Could you check a few things on this model? Use its own coordinates, in mm. Face numbers are marked on the shaded views. Round coordinates to 2 decimals unless told otherwise and drop trailing zeros. Loops run counter-clockwise (first coordinate to the right, second up) from the corner with the lowest first, then second, coordinate; pieces in that order, holes last. Notation, with made-up numbers: (84, 67.5) -> (127, 67.5) arc R28 ccw to (127, 96.5) -> close; hole circle Ø4 at (68, 55.5). An arc over 180 degrees is marked (long way). Write each question's results on one line, items separated by ' | '.
from build123d import *

# Parameters (mm, degrees)
F1_DEPTH = 5
F2_DEPTH = 7
F3_DEPTH = 1


with BuildPart() as f1:
    # F0 (on Top) → F1 (new body)
    with BuildSketch(Plane.XY):
        with BuildLine():
            Line((-12.5, -50), (0, -50))
            Line((0, -50), (0, -45))
            Line((0, -45), (-6.5, -45))
            ThreePointArc((-6.5, -45), (-8.2071067812, -45.7071067812), (-7.5, -44))
            Line((-7.5, -44), (-7.5, -35.9886))
            ThreePointArc((-7.5, -35.9886), (-8.2071067812, -34.2814932188), (-6.5, -34.9886))
            Line((-6.5, -34.9886), (0, -34.9886))
            Line((0, -34.9886), (0, -14.9886))
            Line((0, -14.9886), (-7.5, -14.9886))
            Line((-7.5, -14.9886), (-7.5, -9.9886))
            Line((-7.5, -9.9886), (0, -9.9886))
            Line((0, -9.9886), (0, 0.0114))
            Line((0, 0.0114), (-7.5, 0.0114))
            Line((-7.5, 0.0114), (-7.5, 5.0114))
            Line((-7.5, 5.0114), (0, 5.0114))
            Line((0, 5.0114), (0, 15.0114))
            Line((0, 15.0114), (-7.5, 15.0114))
            Line((-7.5, 15.0114), (-7.5, 20.0114))
            Line((-7.5, 20.0114), (0, 20.0114))
            Line((0, 20.0114), (0, 34.3023235092))
            ThreePointArc((0, 34.3023235092), (-5, 39.3023235092), (0, 44.3023235092))
            Line((0, 44.3023235092), (0, 50))
            Line((0, 50), (-12.5, 50))
            Line((-12.5, 50), (-12.5, -50))
        make_face()
        with BuildLine():
            Line((0, -50), (12.5, -50))
            Line((12.5, -50), (12.5, 50))
            Line((12.5, 50), (0, 50))
            Line((0, 50), (0, 44.3023235092))
            ThreePointArc((0, 44.3023235092), (3.5355339059, 42.8378574152), (5, 39.3023235092))
            ThreePointArc((5, 39.3023235092), (3.5355339059, 35.7667896033), (0, 34.3023235092))
            Line((0, 34.3023235092), (0, 20.0114))
            Line((0, 20.0114), (7.5, 20.0114))
            Line((7.5, 20.0114), (7.5, 15.0114))
            Line((7.5, 15.0114), (0, 15.0114))
            Line((0, 15.0114), (0, 5.0114))
            Line((0, 5.0114), (7.5, 5.0114))
            Line((7.5, 5.0114), (7.5, 0.0114))
            Line((7.5, 0.0114), (0, 0.0114))
            Line((0, 0.0114), (0, -9.9886))
            Line((0, -9.9886), (7.5, -9.9886))
            Line((7.5, -9.9886), (7.5, -14.9886))
            Line((7.5, -14.9886), (0, -14.9886))
            Line((0, -14.9886), (0, -34.9886))
            Line((0, -34.9886), (6.5, -34.9886))
            ThreePointArc((6.5, -34.9886), (7.5, -33.9886), (8.5, -34.9886))
            ThreePointArc((8.5, -34.9886), (8.2071067812, -35.6957067812), (7.5, -35.9886))
            Line((7.5, -35.9886), (7.5, -44))
            ThreePointArc((7.5, -44), (8.2071067812, -44.2928932188), (8.5, -45))
            ThreePointArc((8.5, -45), (7.5, -46), (6.5, -45))
            Line((6.5, -45), (0, -45))
            Line((0, -45), (0, -50))
        make_face()
        with BuildLine():
            Line((0, -34.9886), (0, -45))
            Line((0, -45), (6.5, -45))
            ThreePointArc((6.5, -45), (6.7928932188, -44.2928932188), (7.5, -44))
            Line((7.5, -44), (7.5, -35.9886))
            ThreePointArc((7.5, -35.9886), (6.7928932188, -35.6957067812), (6.5, -34.9886))
            Line((6.5, -34.9886), (0, -34.9886))
        make_face()
        with BuildLine():
            Line((-6.5, -45), (0, -45))
            Line((0, -45), (0, -34.9886))
            Line((0, -34.9886), (-6.5, -34.9886))
            ThreePointArc((-6.5, -34.9886), (-6.7928932188, -35.6957067812), (-7.5, -35.9886))
            Line((-7.5, -35.9886), (-7.5, -44))
            ThreePointArc((-7.5, -44), (-6.7928932188, -44.2928932188), (-6.5, -45))
        make_face()
    extrude(amount=F1_DEPTH)

    # F0 (on Top) → F2 (join)
    with BuildSketch(Plane.XY):
        with BuildLine():
            Line((0, 42.3023235092), (0, 44.3023235092))
            ThreePointArc((0, 44.3023235092), (-5, 39.3023235092), (0, 34.3023235092))
            Line((0, 34.3023235092), (0, 36.3023235092))
            ThreePointArc((0, 36.3023235092), (-3, 39.3023235092), (0, 42.3023235092))
        make_face()
        with BuildLine():
            ThreePointArc((5, 39.3023235092), (3.5355339059, 42.8378574152), (0, 44.3023235092))
            Line((0, 44.3023235092), (0, 42.3023235092))
            ThreePointArc((0, 42.3023235092), (2.1213203436, 41.4236438528), (3, 39.3023235092))
            ThreePointArc((3, 39.3023235092), (2.1213203436, 37.1810031657), (0, 36.3023235092))
            Line((0, 36.3023235092), (0, 34.3023235092))
            ThreePointArc((0, 34.3023235092), (3.5355339059, 35.7667896033), (5, 39.3023235092))
        make_face()
    extrude(amount=F2_DEPTH)

    # F0 (on Top) → F3 (join)
    with BuildSketch(Plane.XY):
        with BuildLine():
            Line((0, 41.8023235092), (0, 42.3023235092))
            ThreePointArc((0, 42.3023235092), (-3, 39.3023235092), (0, 36.3023235092))
            Line((0, 36.3023235092), (0, 36.8023235092))
            ThreePointArc((0, 36.8023235092), (-2.5, 39.3023235092), (0, 41.8023235092))
        make_face()
        with BuildLine():
            ThreePointArc((3, 39.3023235092), (2.1213203436, 41.4236438528), (0, 42.3023235092))
            Line((0, 42.3023235092), (0, 41.8023235092))
            ThreePointArc((0, 41.8023235092), (1.767766953, 41.0700904622), (2.5, 39.3023235092))
            ThreePointArc((2.5, 39.3023235092), (1.767766953, 37.5345565563), (0, 36.8023235092))
            Line((0, 36.8023235092), (0, 36.3023235092))
            ThreePointArc((0, 36.3023235092), (2.1213203436, 37.1810031657), (3, 39.3023235092))
        make_face()
    extrude(amount=F3_DEPTH)


solid = f1.part
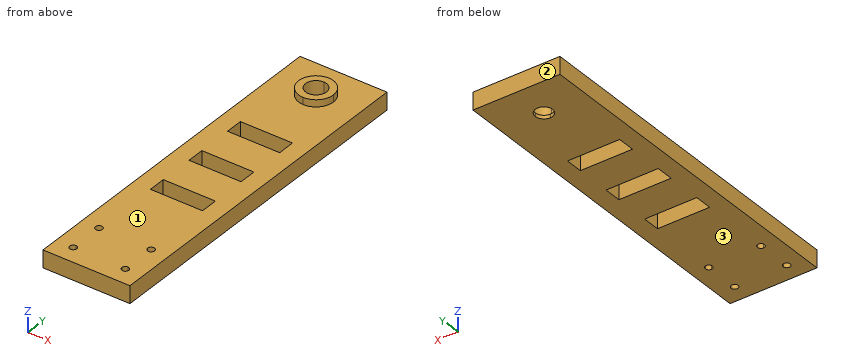
1) I want a section at A-A, the plane y = 19. Write out the boundary of the cut face in (x, z).
Model answer:
outline: (-12.5, 0) -> (-7.5, 0) -> (-7.5, 5) -> (-12.5, 5) -> close; (7.5, 0) -> (12.5, 0) -> (12.5, 5) -> (7.5, 5) -> close
2) I want a section at D-D, the plane y = -6.5. Write out the boundary of the cut face in (x, z).
Model answer:
outline: (-12.5, 0) -> (12.5, 0) -> (12.5, 5) -> (-12.5, 5) -> close
3) If we mould it in two halves opening along Z, with no side actions, what happens to the marked faces 1, 2 and 3? For each: released by +Z, released by -Z, zero draft, split by the parting line, or undercut.
Model answer:
face 1: released by +Z | face 2: zero draft | face 3: released by -Z
4) I want a section at B-B, the plane x = 4. Write out the boundary of the cut face in (y, z), plus the area to 3 significant figures.
Model answer:
outline: (-50, 0) -> (-14.99, 0) -> (-14.99, 5) -> (-50, 5) -> close; (-9.99, 0) -> (0.01, 0) -> (0.01, 5) -> (-9.99, 5) -> close; (5.01, 0) -> (15.01, 0) -> (15.01, 5) -> (5.01, 5) -> close; (20.01, 0) -> (50, 0) -> (50, 5) -> (42.3, 5) -> (42.3, 7) -> (36.3, 7) -> (36.3, 5) -> (20.01, 5) -> close | area: 437 mm2
5) I need wall thicknesses on line 1 (Y direction, x = -5, z = 3.75); line 2 (X direction, y = 17.5, z = 4.25); line 3 (Z direction, x = -6.25, y = 13). Which ranges of each line are inside material? Lowest first, please.
Model answer:
line 1: y = -50 to -14.99, -9.99 to 0.01, 5.01 to 15.01, 20.01 to 50 | line 2: x = -12.5 to -7.5, 7.5 to 12.5 | line 3: z = 0 to 5
6) I want a section at C-C, the plane x = 10. Write out the boundary of the cut face in (y, z).
Model answer:
outline: (-50, 0) -> (50, 0) -> (50, 5) -> (-50, 5) -> close
7) I'm going to push a flat-ended pin straight in: pin 1 (5 mm diameter, centred on x = 8.5, y = -30, fed in from +Z). Where does the tip first touch, or does it pass through?
Model answer:
pin 1: stops at z = 5
